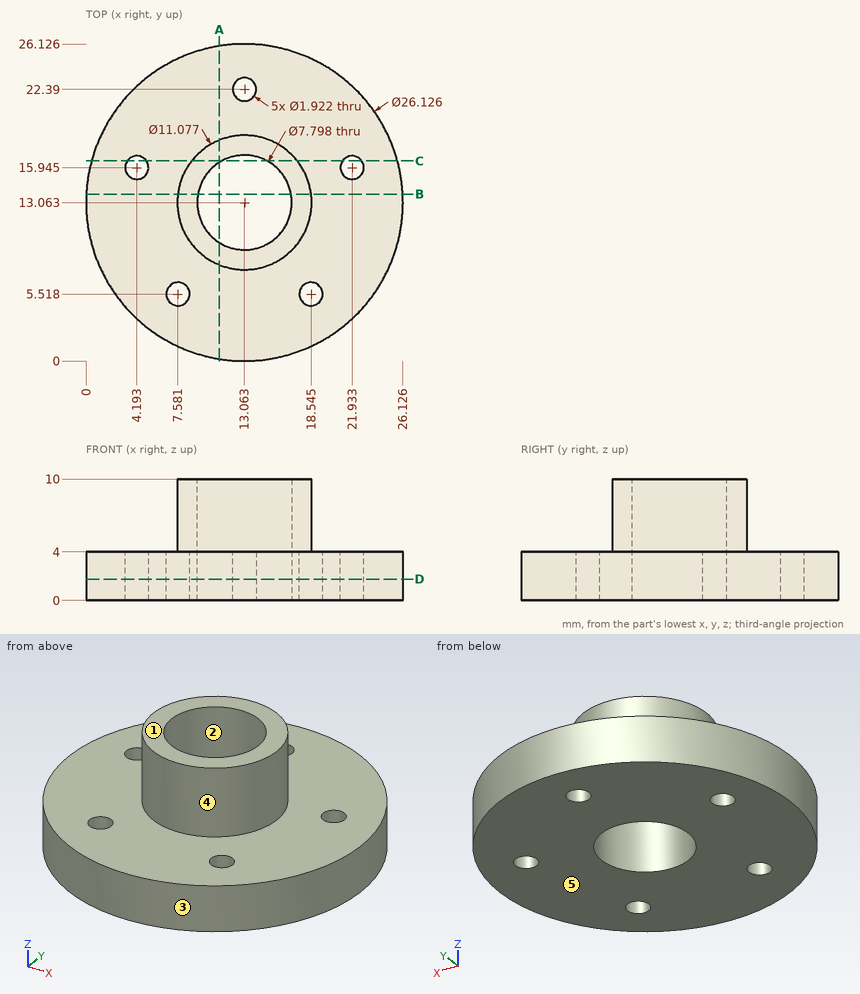
Verification items for this drawing (mm, ordinates from the low corner). A direction names the side the tool comes from. Coordinates: 2 decimals unless noted, no trailing zeros. Loops run counter-clockwise (first coordinate to the right, second up) from the corner with the lowest first, then second, coordinate; pieces in that order, holes last. Notation, with made-up numbers: (28.5, 87.25) -> (62.5, 87.25) arc R27 ccw to (62.5, 124.25) -> close; hole circle Ø11 at (23.5, 82.25). An arc over 180 degrees is marked (long way). Put each result on its own line as item: value.
1. Section check D-D, the plane z = 1.75. Record the boundary of the cut face in (x, y) (1 decimal).
Result set:
outline: circle Ø26.1 at (13.1, 13.1); hole circle Ø1.9 at (4.2, 15.9); hole circle Ø1.9 at (7.6, 5.5); hole circle Ø7.8 at (13.1, 13.1); hole circle Ø1.9 at (13.1, 22.4); hole circle Ø1.9 at (18.5, 5.5); hole circle Ø1.9 at (21.9, 15.9)
2. Mould release check, pull along Y, two halves, no side actions. Record for the marked faces 1, 2 and 3: pulls with the +Y half, pulls with the -Y half, needs draft (parallel to the pull), parting line crosses it, or undercut.
Result set:
face 1: needs draft
face 2: undercut
face 3: parting line crosses it
3. Thickness scan on line 1 (Z direction, x = 19.5, y = 12.25); line 2 (X direction, y = 14.25, z = 6.5); line 3 (Y direction, x = 18.25, z = 1.25) (1 decimal). Record the ranges inside material, lowest first.
Result set:
line 1: z = 0 to 4
line 2: x = 7.65 to 9.35, 16.78 to 18.47
line 3: y = 1.1 to 4.6, 6.4 to 25.1
4. Gauge pin test, flat ends, axial feed: P1, Ø1.2, axis at x = 13.06, y = 22.39, coming from the +Z side; P2, Ø2.5, axis at x = 4.19, y = 15.95, coming from the +Z side; P3, Ø3, axis at x = 8.5, z = 4, coming from the +Y side; P4, Ø2, axis at y = 8.5, z = 8.5, coming from the +X side (1 decimal). Record the tip position at first contact, or that the pin passes through.
Result set:
P1: passes through
P2: stops at z = 4
P3: stops at y = 25.76
P4: stops at x = 17.3
5. Section check B-B, the plane y = 13.75. Record the boundary of the cut face in (x, z) (1 decimal).
Result set:
outline: (0, 0) -> (9.2, 0) -> (9.2, 10) -> (7.6, 10) -> (7.6, 4) -> (0, 4) -> close; (16.9, 0) -> (26.1, 0) -> (26.1, 4) -> (18.6, 4) -> (18.6, 10) -> (16.9, 10) -> close
6. Section check A-A, the plane x = 11. Record the boundary of the cut face in (y, z) (1 decimal).
Result set:
outline: (0.2, 0) -> (9.8, 0) -> (9.8, 10) -> (7.9, 10) -> (7.9, 4) -> (0.2, 4) -> close; (16.4, 0) -> (26, 0) -> (26, 4) -> (18.2, 4) -> (18.2, 10) -> (16.4, 10) -> close
7. Section check C-C, the plane y = 16.5. Record the boundary of the cut face in (x, z) (1 decimal).
Result set:
outline: (0.5, 0) -> (3.4, 0) -> (3.4, 4) -> (0.5, 4) -> close; (5, 0) -> (11.2, 0) -> (11.2, 10) -> (8.7, 10) -> (8.7, 4) -> (5, 4) -> close; (14.9, 0) -> (21.1, 0) -> (21.1, 4) -> (17.4, 4) -> (17.4, 10) -> (14.9, 10) -> close; (22.7, 0) -> (25.7, 0) -> (25.7, 4) -> (22.7, 4) -> close
8. Tool access check on the marked faces 4 and 5. Record the directions out of +Z, -Z, +X, -X, +Y, -Y that give a thin tool (end or side, any length) a straight path to the whole face; none if there is none.
Result set:
face 4: +Z
face 5: -Z, +X, -X, +Y, -Y
